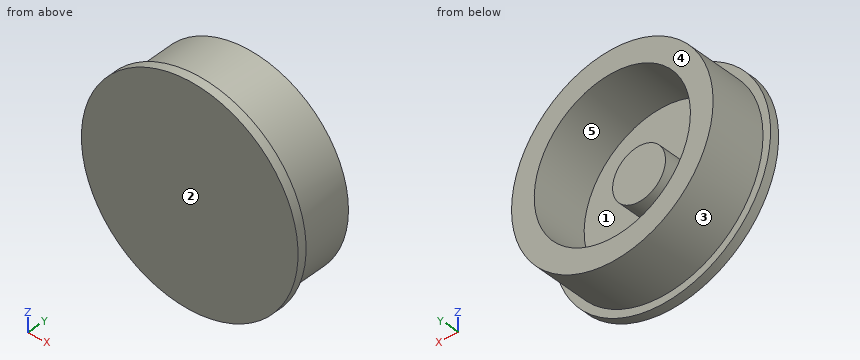
from build123d import *

# Parameters (mm, degrees)
F_01_BOWL_FLANGE_PROFILE_R   = 215
F_01_BOWL_FLANGE_PROFILE_R_2 = 6
F_01_BOWL_BASE_FLANGE_DEPTH  = 18
F_02_BOWL_WALL_PROFILE_R     = 200
F_02_BOWL_WALL_PROFILE_R_2   = 155
F_02_BOWL_WALL_DEPTH         = 130
F_03_CENTER_CONE_BASE_R      = 52.5
F_03_CENTER_GUIDE_BOSS_DEPTH = 70


with BuildPart() as part:
    # 01_Bowl_Flange_Profile → 01_Bowl_Base_Flange (new body)
    with BuildSketch(Plane(origin=(0, 0, 0), x_dir=(1, 0, 0), z_dir=(0, 1, 0))):
        with Locations(Location((0, 0, 0), (0, 0, 270))):
            Circle(F_01_BOWL_FLANGE_PROFILE_R)
        with Locations(Location((170.917713515, 70.796434988, 0), (0, 0, 270))):
            Circle(F_01_BOWL_FLANGE_PROFILE_R_2, mode=Mode.SUBTRACT)
        with Locations(Location((70.796434988, 170.917713515, 0), (0, 0, 270))):
            Circle(F_01_BOWL_FLANGE_PROFILE_R_2, mode=Mode.SUBTRACT)
        with Locations(Location((-70.796434988, 170.917713515, 0), (0, 0, 270))):
            Circle(F_01_BOWL_FLANGE_PROFILE_R_2, mode=Mode.SUBTRACT)
        with Locations(Location((-170.917713515, 70.796434988, 0), (0, 0, 270))):
            Circle(F_01_BOWL_FLANGE_PROFILE_R_2, mode=Mode.SUBTRACT)
        with Locations(Location((-170.917713515, -70.796434988, 0), (0, 0, 270))):
            Circle(F_01_BOWL_FLANGE_PROFILE_R_2, mode=Mode.SUBTRACT)
        with Locations(Location((-70.796434988, -170.917713515, 0), (0, 0, 270))):
            Circle(F_01_BOWL_FLANGE_PROFILE_R_2, mode=Mode.SUBTRACT)
        with Locations(Location((70.796434988, -170.917713515, 0), (0, 0, 270))):
            Circle(F_01_BOWL_FLANGE_PROFILE_R_2, mode=Mode.SUBTRACT)
        with Locations(Location((170.917713515, -70.796434988, 0), (0, 0, 270))):
            Circle(F_01_BOWL_FLANGE_PROFILE_R_2, mode=Mode.SUBTRACT)
    extrude(amount=F_01_BOWL_BASE_FLANGE_DEPTH)

    # 02_Bowl_Wall_Profile → 02_Bowl_Wall (add)
    with BuildSketch(Plane(origin=(0, 0, 0), x_dir=(1, 0, 0), z_dir=(0, 1, 0))):
        with Locations(Location((0, 0, 0), (0, 0, 270))):
            Circle(F_02_BOWL_WALL_PROFILE_R)
        with Locations(Location((0, 0, 0), (0, 0, 270))):
            Circle(F_02_BOWL_WALL_PROFILE_R_2, mode=Mode.SUBTRACT)
    extrude(amount=F_02_BOWL_WALL_DEPTH)

    # 03_Center_Cone_Base → 03_Center_Guide_Boss (add)
    with BuildSketch(Plane(origin=(0, 0, 0), x_dir=(1, 0, 0), z_dir=(0, 1, 0))):
        with Locations(Location((0, 0, 0), (0, 0, 270))):
            Circle(F_03_CENTER_CONE_BASE_R)
    extrude(amount=F_03_CENTER_GUIDE_BOSS_DEPTH)


solid = part.part
Can you work these out from the model? Positions are in its coordinate system, mm. Face numbers are marked on the shaded views. A direction names the side the tool comes from. Give positions to 0.01 mm unless a question says otherwise; leave off trailing zeros. Order: outer loops, then holes, each group sorted by start corner. A loop starts at its lowest first (then second) coordinate and runs counter-clockwise, first axis right, second up. Notation, with made-up numbers: M -30,27 L 7,27 A16 cw 7,48 Z; hole C -16,89.25 d3. An arc over 180 degrees is marked long. One line per item, written item: value.
Item 1: If we section it at B-B on x = 0: Write out the boundary of the cut face in (y, z).
Verdict:
outline: M 0,-215 L 18,-215 L 18,-200 L 130,-200 L 130,-155 L 18,-155 L 18,-52.5 L 70,-52.5 L 70,52.5 L 18,52.5 L 18,155 L 130,155 L 130,200 L 18,200 L 18,215 L 0,215 Z
Item 2: For the marked faces 4 and 5, which set-ups out of +Z, -Z, +X, -X, +Y, -Y let a thin tool reach every point of the face, with its end or its side?
Verdict:
face 4: +Z, -Z, +X, -X, +Y
face 5: +Y
Item 3: If we section it at D-D on y = 10.5: Write out the boundary of the cut face in (x, z).
Verdict:
outline: C 0,0 d430
Item 4: If we section it at A-A on z = 0: Write out the boundary of the cut face in (x, y).
Verdict:
outline: M -215,0 L 215,0 L 215,18 L 200,18 L 200,130 L 155,130 L 155,18 L 52.5,18 L 52.5,70 L -52.5,70 L -52.5,18 L -155,18 L -155,130 L -200,130 L -200,18 L -215,18 Z
Item 5: If we mould it in two halves opening along Z, with no side actions, what happens to the marked faces 1, 2 and 3? For each: pulls with the +Z half, pulls with the -Z half, needs draft (parallel to the pull), parting line crosses it, or undercut.
Verdict:
face 1: undercut
face 2: needs draft
face 3: parting line crosses it
Item 6: If we section it at C-C on y = 85: Write out the boundary of the cut face in (x, z).
Verdict:
outline: C 0,0 d400; hole C 0,0 d310
Item 7: For pin 1 (3 mm diameter, centred on y = 73, z = 23, fed in from -X); pin 2 (12 mm diameter, centred on y = 33.5, z = -73, fed in from -X); pin 3 (2 mm diameter, centred on y = 51.5, z = -142, fed in from -X), each with a flat end and sliding along its axis, tell me the tip position at first contact or that it passes through.
Verdict:
pin 1: x = -198.84
pin 2: x = -188.44
pin 3: x = -141.84
Item 8: Please list where these lines run through material, in increasing order: line 1 (Z direction, x = 0, y = 59); line 2 (Z direction, x = 0, y = 96.5).
Verdict:
line 1: -200 to -155, -52.5 to 52.5, 155 to 200
line 2: -200 to -155, 155 to 200
